Design review of the part built by this model. Coordinates are the model's own, in mm. A direction names the side the tool comes from. Round coordinates to 2 decimals unless told otherwise and drop trailing zeros. Write each loop counter-clockwise with the first axis right and the second up, starting at its lowest first coordinate (ties: lowest second). Pieces come first, ordered by that corner, then holes. Notation, with made-up numbers: M 11.5,38 L 25.5,38 A14 ccw 25.5,64 Z; hole C -6,47.5 d2. An arc over 180 degrees is marked long. Use CSV: the item, a comma, the result in double quotes.
from build123d import *

# Parameters (mm, degrees)
F1_DEPTH = 25.4
F3_DEPTH = 19.05
F5_DEPTH = 19.05


with BuildPart() as f1:
    # F0 (on Front) → F1 (new body, symmetric)
    with BuildSketch(Plane.XZ):
        Polygon((0, 0), (0, 2.3114), (-28.900176, 22.547521), (-84.703976, 22.547521), (-84.703976, -15.298479), (-51.210209, -63.132535), (-48.898809, -63.132535), (-48.898809, -67.348935), (-51.210209, -67.348935), (-84.703976, -115.182991), (-84.703976, -165.322591), (-37.434576, -165.322591), (-2.503217, -138.999924), (-2.503217, -136.688524), (0.702485, -136.679767), (0.702485, -138.991167), (36.748776, -163.765096), (87.066176, -163.765096), (87.066176, -117.994296), (52.55259, -68.703787), (50.24119, -68.703787), (50.24119, -64.487387), (52.55259, -64.487387), (87.066176, -15.196879), (87.066176, 22.547521), (33.116576, 22.547521), (4.2164, 2.3114), (4.2164, 0), align=None)
    extrude(amount=F1_DEPTH, both=True)

    # F2 (on face) → F3 (cut)
    with BuildSketch(Plane.XZ.offset(25.4)):
        Polygon((-18.251217, -120.983487), (16.450485, -120.888687), (16.450485, -130.705743), (41.63866, -148.017096), (71.318176, -148.017096), (71.318176, -122.959621), (44.3547, -84.451787), (34.49319, -84.451787), (34.49319, -48.739387), (44.3547, -48.739387), (71.318176, -10.231554), (71.318176, 6.799521), (38.081901, 6.799521), (19.9644, -5.88649), (19.9644, -15.748), (-15.748, -15.748), (-15.748, -5.88649), (-33.865501, 6.799521), (-68.955976, 6.799521), (-68.955976, -10.333154), (-43.012319, -47.384535), (-33.150809, -47.384535), (-33.150809, -83.096935), (-43.012319, -83.096935), (-68.955976, -120.148316), (-68.955976, -149.574591), (-42.703783, -149.574591), (-18.251217, -131.148261), align=None)
    extrude(amount=-F3_DEPTH, mode=Mode.SUBTRACT)

    # F4 (on face) → F5 (cut)
    with BuildSketch(Plane(origin=(0, 25.4, 0), x_dir=(-1, 0, 0), z_dir=(0, 1, 0))):
        Polygon((-71.318176, -122.959621), (-71.318176, -148.017096), (-41.63866, -148.017096), (-16.450485, -130.705743), (-16.450485, -120.888687), (18.251217, -120.983487), (18.251217, -131.148261), (42.703783, -149.574591), (68.955976, -149.574591), (68.955976, -120.148316), (43.012319, -83.096935), (33.150809, -83.096935), (33.150809, -47.384535), (43.012319, -47.384535), (68.955976, -10.333154), (68.955976, 6.799521), (33.865501, 6.799521), (15.748, -5.88649), (15.748, -15.748), (-19.9644, -15.748), (-19.9644, -5.88649), (-38.081901, 6.799521), (-71.318176, 6.799521), (-71.318176, -10.231554), (-44.3547, -48.739387), (-34.49319, -48.739387), (-34.49319, -84.451787), (-44.3547, -84.451787), align=None)
    extrude(amount=-F5_DEPTH, mode=Mode.SUBTRACT)


solid = f1.part
1) Add section D-D on x = -21. Write out the cut boundary in (y, z).
Answers:
outline,"M -25.4,-152.94 L 25.4,-152.94 L 25.4,-133.22 L 6.35,-133.22 L 6.35,-2.21 L 25.4,-2.21 L 25.4,17.02 L -25.4,17.02 L -25.4,-2.21 L -6.35,-2.21 L -6.35,-133.22 L -25.4,-133.22 Z"
2) Add section C-C on z = -73. Write out the cut boundary in (x, y).
Answers:
outline,"M -55.17,-25.4 L -33.15,-25.4 L -33.15,-6.35 L 34.49,-6.35 L 34.49,-25.4 L 55.56,-25.4 L 55.56,25.4 L 34.49,25.4 L 34.49,6.35 L -33.15,6.35 L -33.15,25.4 L -55.17,25.4 Z"
3) Wall thickness on line 1 along X through (y, z) = (-9, -130); line 2 along Z through (x, y) = (-50.5, 23); line 3 along Z through (x, y) = (-41, -16): over which ranges is each line inside the solid? List them lowest first. Write a range as [from, to].
Answers:
line 1,"[-84.7, -68.96], [-18.25, 16.45], [71.32, 87.07]"
line 2,"[-165.32, -149.57], [-93.79, -67.35], [-63.13, -36.69], [6.8, 22.55]"
line 3,"[-165.32, -148.29], [-83.1, -47.38], [6.8, 22.55]"
4) Add section B-B on y = 1.5. Write out the cut boundary in (x, z), then the cut area to 3 significant figures.
Answers:
outline,"M -84.7,-165.32 L -37.43,-165.32 L -2.5,-139 L -2.5,-136.69 L 0.7,-136.68 L 0.7,-138.99 L 36.75,-163.77 L 87.07,-163.77 L 87.07,-117.99 L 52.55,-68.7 L 50.24,-68.7 L 50.24,-64.49 L 52.55,-64.49 L 87.07,-15.2 L 87.07,22.55 L 33.12,22.55 L 4.22,2.31 L 4.22,0 L 0,0 L 0,2.31 L -28.9,22.55 L -84.7,22.55 L -84.7,-15.3 L -51.21,-63.13 L -48.9,-63.13 L -48.9,-67.35 L -51.21,-67.35 L -84.7,-115.18 Z"
area,"26,800 mm²"
5) The part is to be moulded in two halves that separate along Z. For faces 1 (the face through (-33.151, -16, -65)), 2 (the face through (60, 0, 22.548)), 3 (the face through (55, -16, 6.8)), say which applies: released by +Z, released by -Z, zero draft, split by the parting line, or undercut.
Answers:
face 1,"undercut"
face 2,"released by +Z"
face 3,"undercut"
6) Machinability: for faces 4 (the face through (69.568, -0.356, -40.187)), 5 (the face through (-24.68, -16.01, 0.37)), 6 (the face through (-68.956, 16, -2)), 7 (the face through (-48.899, 0, -65)), which of the approach directions +Z, -Z, +X, -X, +Y, -Y give a long, thin tool a straight path to every point of the face, cutting with its end or side? Answer none if there is none.
Answers:
face 4,"+X, +Y, -Y"
face 5,"-Y"
face 6,"+Y"
face 7,"-X, +Y, -Y"
7) For pin 1 Ø15 at (x, y) = (55, -12) entering from -Z; pin 2 Ø4 at (y, z) = (-18, -93.5) entering from -X; pin 3 Ø6 at (x, z) = (12.5, -55) entering from -Y, all flat-tipped, find the tip position at first contact; note any pin that passes through.
Answers:
pin 1,"z = -163.77"
pin 2,"x = -70.92"
pin 3,"y = -6.35"
8) Add section A-A on x = 60. Write out the cut boundary in (y, z), then the cut area to 3 significant figures.
Answers:
outline,"M -25.4,-163.77 L 25.4,-163.77 L 25.4,-148.02 L 6.35,-148.02 L 6.35,-106.8 L 25.4,-106.8 L 25.4,-79.34 L -25.4,-79.34 L -25.4,-106.8 L -6.35,-106.8 L -6.35,-148.02 L -25.4,-148.02 Z; M -25.4,-53.85 L 25.4,-53.85 L 25.4,-26.4 L 6.35,-26.4 L 6.35,6.8 L 25.4,6.8 L 25.4,22.55 L -25.4,22.55 L -25.4,6.8 L -6.35,6.8 L -6.35,-26.4 L -25.4,-26.4 Z"
area,"5,330 mm²"
